Here's how the part is built. I have some questions about the finished solid (model axes, mm). Face numbers are marked on the shaded views. A direction names the side the tool comes from. Coordinates: 2 decimals unless noted, no trailing zeros. Write each loop counter-clockwise with the first axis right and the second up, starting at its lowest first coordinate (ties: lowest second). Pieces come first, ordered by that corner, then holes.
Item 1: I want a section at D-D (z = 8.25). Please give me the cut outline in (x, y).
Item 2: If we mould it in two halves opening along Y, with no side actions, what happens to the marked faces 3, 4 and 5? For each: pulls with the +Y half, pulls with the -Y half, needs draft (parallel to the pull), parting line crosses it, or undercut.
Item 3: Please list where these lines run through material, in increasing order: line 1 (Y direction, x = 12, z = 2.6); line 2 (Z direction, x = 9.75, y = 18); line 3 (Z direction, x = 2.5, y = 5.25).
Item 4: For the marked faces 1 and 2, which set-ups out of +Z, -Z, +X, -X, +Y, -Y let a thin tool reach every point of the face, with its end or its side?
Item 5: I'm going to push a flat-ended pin straight in: P1, Ø4, axis at x = 4.5, y = 9, coming from the +Z side. Where does the tip first touch, or does it pass through?
Item 6: I want a section at B-B (z = 4.75). Please give me the cut outline in (x, y).
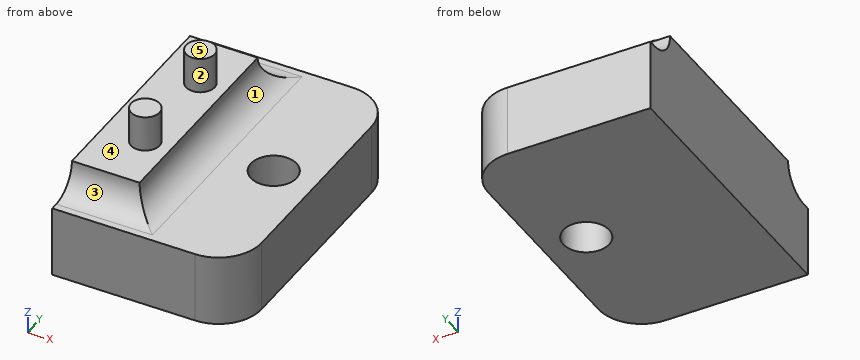
from build123d import *

# Parameters (mm, degrees)
CROQUIS1_R                 = 1.6
SALIENTE_EXTRUIR1_DEPTH    = 5
CROQUIS2_W                 = 6.75
CROQUIS2_H                 = 15
SALIENTE_EXTRUIR2_DEPTH    = 2
REDONDEO1_R                = 2
CROQUIS3_R                 = 1
SALIENTE_EXTRUIR3_DEPTH    = 2.5
CORTAR_EXTRUIR2_DEPTH      = 6
CORTAR_EXTRUIR2_DEPTH_BACK = 6
CROQUIS4_W                 = 6.920457475
CROQUIS4_H                 = 24.995599696


with BuildPart() as part:
    # Croquis1 → Saliente-Extruir1 (new body)
    with BuildSketch(Plane.XY):
        with BuildLine():
            Line((0, 0), (12, 0))
            ThreePointArc((12, 0), (14.121320344, 0.878679656), (15, 3))
            Line((15, 3), (15, 17))
            ThreePointArc((15, 17), (14.121320344, 19.121320344), (12, 20))
            Line((12, 20), (0, 20))
            Line((0, 20), (0, 0))
        make_face()
        with Locations((12, 10)):
            Circle(CROQUIS1_R, mode=Mode.SUBTRACT)
    extrude(amount=SALIENTE_EXTRUIR1_DEPTH)

    # Croquis2 → Saliente-Extruir2 (add)
    with BuildSketch(Plane.XY.offset(5)):
        with Locations((3.375, 10)):
            Rectangle(CROQUIS2_W, CROQUIS2_H)
    extrude(amount=SALIENTE_EXTRUIR2_DEPTH)

    # Redondeo1
    redondeo1_edges = [part.edges().sort_by_distance(p)[0] for p in [
        (3.375, 17.5, 5),
        (6.75, 10, 5),
        (3.375, 2.5, 5),
    ]]
    fillet(redondeo1_edges, radius=REDONDEO1_R - 0.0001)  # a hair under: the kernel refuses the full size

    # Croquis3 → Saliente-Extruir3 (add)
    with BuildSketch(Plane.XY.offset(7)):
        with Locations((4.95023571, 13.5)):
            Circle(CROQUIS3_R)
        with Locations((4.95023571, 6.5)):
            Circle(CROQUIS3_R)
    extrude(amount=SALIENTE_EXTRUIR3_DEPTH)

    # Croquis4 → Cortar-Extruir2 (cut, two sides: drawn at the far end of the back side and taken through both)
    with BuildSketch(Plane.XY.offset(5).offset(-CORTAR_EXTRUIR2_DEPTH_BACK)):
        with Locations((-1.442627952, 9.887678484)):
            Rectangle(CROQUIS4_W, CROQUIS4_H)
    extrude(amount=CORTAR_EXTRUIR2_DEPTH + CORTAR_EXTRUIR2_DEPTH_BACK, mode=Mode.SUBTRACT)


solid = part.part
Answer:
1. outline: circle Ø2 at (4.95, 6.5); circle Ø2 at (4.95, 13.5)
2. face 3: pulls with the -Y half
2. face 4: undercut
2. face 5: needs draft
3. line 1: y = 0 to 8.4, 11.6 to 20
3. line 2: z = 0 to 5
3. line 3: z = 0 to 7
4. face 1: +Z, +X, +Y, -Y
4. face 2: +Z
5. P1: stops at z = 9.5
6. outline: (2.02, 0) - (12, 0) arc R3 ccw to (15, 3) - (15, 17) arc R3 ccw to (12, 20) - (2.02, 20) - close; hole circle Ø3.2 at (12, 10)
